Input: part model. Units: mm. Frame: model coordinates. Face numbers are marked on the shaded views. A direction names the side the tool comes from. Give positions to 0.01 mm unless a question says otherwise; leave off trailing zeros. Loops run counter-clockwise (first coordinate to the right, second up) from the corner with the lowest first, then second, coordinate; pieces in that order, holes last. Notation, with made-up numbers: (23, 66) -> (28, 66) arc R23 cw to (28, 91) -> close; hole circle Ø1 at (11, 34.5). An arc over 180 degrees is marked (long way). Use CSV: the item, a comma, the result in double quotes.
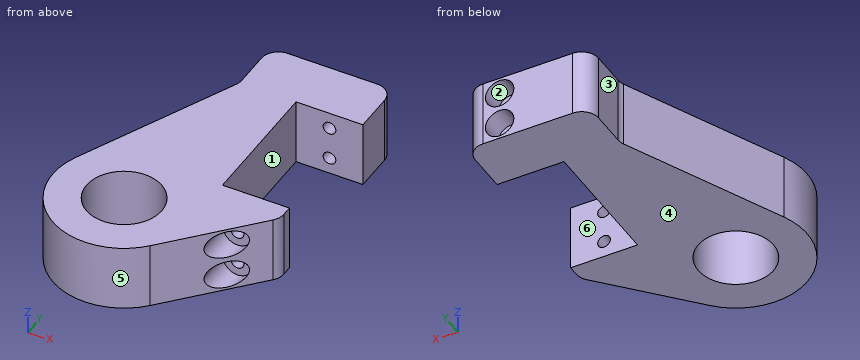
```python
from build123d import *

# Parameters (mm, degrees)
SKETCH1_R               = 14.2875
INITIAL_PLATE_DEPTH     = 25.4
INITIAL_START           = -22.347989325
SKETCH3_R               = 2.413
INITIAL_BOLT_HOLE_DEPTH = 122.882919484
INITIAL_START_2         = -12.7
SKETCH3_3_R             = 5.3975
SKETCH3_3_R_2           = 2.413
INITIAL_HEAD_HOLE_DEPTH = 9.647989325
OTHER_START             = 90.807702
SKETCH3_4_R             = 5.3975
SKETCH3_4_R_2           = 2.413
OTHER_HEAD_HOLE_DEPTH   = 27.307702
MOUNTING_PATTERN_COUNT  = 2
MOUNTING_PATTERN_PITCH  = 12.7
FILLET1_R               = 6.35


with BuildPart() as part:
    # Sketch1 → Initial Plate (new body)
    with BuildSketch(Plane(origin=(0, -13.010095613, 793.75), x_dir=(1, 0, 0), z_dir=(0, 0, 1))):
        with BuildLine():
            Line((-3.175, -125.901852304), (-28.575, -125.901852304))
            Line((-28.575, -125.901852304), (-28.575, -75.101852304))
            Line((-28.575, -75.101852304), (-3.175, -75.101852304))
            Line((-3.175, -75.101852304), (-3.175, -53.753862978))
            Line((-3.175, -53.753862978), (-49.922989325, -53.753862978))
            Line((-49.922989325, -53.753862978), (-49.922989325, -75.101852304))
            Line((-49.922989325, -75.101852304), (-78.433981403, -136.243872124))
            ThreePointArc((-78.433981403, -136.243872124), (-68.984123144, -170.078089357), (-34.103220183, -165.909554179))
            Line((-34.103220183, -165.909554179), (-3.175, -132.251852304))
            Line((-3.175, -132.251852304), (-3.175, -125.901852304))
        make_face()
        with Locations((-53.975, -147.649282463)):
            Circle(SKETCH1_R, mode=Mode.SUBTRACT)
    extrude(amount=INITIAL_PLATE_DEPTH)

    # Sketch3 → Initial Bolt Hole (cut)
    with BuildSketch(Plane.XZ.offset(88.111947917).offset(INITIAL_START)):
        with Locations((-15.875, 800.1)):
            Circle(SKETCH3_R)
    initial_bolt_hole = extrude(amount=INITIAL_BOLT_HOLE_DEPTH, mode=Mode.SUBTRACT)

    # Sketch3<3> → Initial Head Hole (cut, through all)
    with BuildSketch(Plane.XZ.offset(88.111947917).offset(INITIAL_START_2)):
        with Locations((-15.875, 800.1)):
            Circle(SKETCH3_3_R)
        with Locations((-15.875, 800.1)):
            Circle(SKETCH3_3_R_2, mode=Mode.SUBTRACT)
    initial_head_hole = extrude(amount=-INITIAL_HEAD_HOLE_DEPTH, mode=Mode.SUBTRACT)

    # Sketch3<4> → Other Head Hole (cut)
    with BuildSketch(Plane.XZ.offset(88.111947917).offset(OTHER_START)):
        with Locations((-15.875, 800.1)):
            Circle(SKETCH3_4_R)
        with Locations((-15.875, 800.1)):
            Circle(SKETCH3_4_R_2, mode=Mode.SUBTRACT)
    other_head_hole = extrude(amount=-OTHER_HEAD_HOLE_DEPTH, mode=Mode.SUBTRACT)

    # Mounting Pattern: Initial Bolt Hole, Initial Head Hole, Other Head Hole ×2
    with Locations(*[(0, 0, i * MOUNTING_PATTERN_PITCH) for i in range(1, MOUNTING_PATTERN_COUNT)]):
        add(initial_bolt_hole, mode=Mode.SUBTRACT)
        add(initial_head_hole, mode=Mode.SUBTRACT)
        add(other_head_hole, mode=Mode.SUBTRACT)

    # Fillet1
    fillet1_edges = [part.edges().sort_by_distance(p)[0] for p in [
        (-3.175, -145.261947917, 806.45),
        (-49.922989325, -88.111947917, 806.45),
        (-49.922989325, -66.763958592, 806.45),
        (-3.175, -66.763958592, 806.45),
    ]]
    fillet(fillet1_edges, radius=FILLET1_R)


solid = part.part
```
1) Ray query, line 1 (X direction, y = -148.25, z = 800.1); line 2 (X direction, y = -73.5, z = 800.1) (1 decimal); line 3 (Z direction, x = -18, y = -86). Return the intervals inside material, ascending.
From the geometry:
line 1,"x = -77.97 to -61.06, -46.89 to -18.29, -13.46 to -5.92"
line 2,"x = -49.9 to -21.3, -10.5 to -3.2"
line 3,"z = 793.75 to 798.96, 801.24 to 811.66, 813.94 to 819.15"
2) Contact query for flat-ended pins moving along their axis: pin 1 (12 mm diameter, centred on x = -31.5, z = 805.5, fed in from -Y); pin 2 (8.5 mm diameter, centred on x = -14.5, z = 813.5, fed in from +Y); pin 3 (1 mm diameter, centred on x = -68.5, z = 803.5, fed in from +Y); pin 4 (3 mm diameter, centred on x = -36.5, z = 799, fed in from -Y). Output: stop coordinate, or through.
From the geometry:
pin 1,"stops at y = -182.03"
pin 2,"stops at y = -66.76"
pin 3,"stops at y = -126.88"
pin 4,"stops at y = -182.41"
3) Section query C-C (x = -8). Return loops of the section in (y, z).
From the geometry:
outline,"(-150.51, 793.75) -> (-138.91, 793.75) -> (-138.91, 819.15) -> (-150.51, 819.15) -> close; (-88.11, 793.75) -> (-66.95, 793.75) -> (-66.95, 819.15) -> (-88.11, 819.15) -> close"
4) Reachability of the marked faces 1, 2 and 3 from +Z, -Z, +X, -X, +Y, -Y: full face, straight path, thin tool, end or side. Return the list, or none.
From the geometry:
face 1,"+Z, -Z, +X"
face 2,"+Y"
face 3,"+Z, -Z, -X, +Y"
5) Section query D-D (x = -37.5). Return loops of the section in (y, z).
From the geometry:
outline,"(-182.03, 793.75) -> (-66.76, 793.75) -> (-66.76, 819.15) -> (-182.03, 819.15) -> close"
6) Mould query, pull axis Y, two halves, no side actions, for the marked faces 4, 5 and 6. Classes: pulls with the +Y half, pulls with the -Y half, needs draft (parallel to the pull), parting line crosses it, or undercut.
From the geometry:
face 4,"needs draft"
face 5,"parting line crosses it"
face 6,"undercut"
7) Section query B-B (x = -60.5). Return loops of the section in (y, z), then the cut area to 3 significant figures.
From the geometry:
outline,"(-186.85, 793.75) -> (-173.37, 793.75) -> (-173.37, 819.15) -> (-186.85, 819.15) -> close; (-147.95, 793.75) -> (-110.79, 793.75) -> (-110.79, 819.15) -> (-147.95, 819.15) -> close"
area,"1,290 mm^2"
8) Section query A-A (z = 800.1). Give the number of separate pieces and of enclosed holes in the cut face, then the cut area to 3 significant figures.
From the geometry:
separate pieces,"3"
enclosed holes,"1"
area,"4,460 mm^2"
